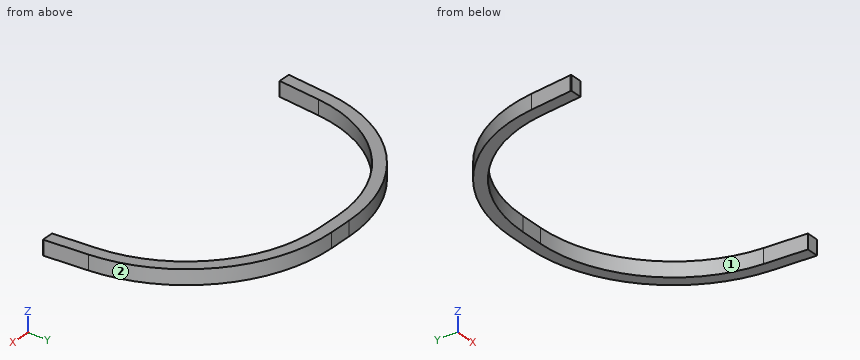
from build123d import *

# Parameters (mm, degrees)
EXTRUDE_1_DEPTH      = 5
SKETCH_3_W           = 25
SKETCH_3_H           = 3
SKETCH_3_W_2         = 27.5
CUT_EXTRUDE_1_DEPTH  = 396.82192966
SKETCH_2_R           = 1
CUT_EXTRUDE_2_DEPTH  = 396.82192966
SKETCH_4_R           = 1
CUT_EXTRUDE_3_DEPTH  = 396.82192966
SKETCH_5_W           = 3
SKETCH_5_H           = 20
CUT_EXTRUDE_4_DEPTH  = 396.82192966
SKETCH_6_W           = 52.963954937
SKETCH_6_H           = 5
SKETCH_6_W_2         = 50.247879271
CUT_EXTRUDE_5_DEPTH  = 396.82192966
SKETCH_7_W           = 24.499878537
SKETCH_7_H           = 5
SKETCH_7_W_2         = 25.63433041
SKETCH_7_W_3         = 30.65568147
SKETCH_7_W_4         = 13.75
CUT_EXTRUDE_6_DEPTH  = 396.82192966
CUT_EXTRUDE_10_DEPTH = 396.82192966
SKETCH_12_W          = 10
SKETCH_12_H          = 114.036005351
CUT_EXTRUDE_11_DEPTH = 396.82192966
SKETCH_13_W          = 5
SKETCH_13_H          = 15
EXTRUDE_2_DEPTH      = 3
CUT_EXTRUDE_12_DEPTH = 396.82192966
FILLET_1_R           = 45
CUT_EXTRUDE_13_DEPTH = 396.82192966


with BuildPart() as part:
    # 草图1 → 凸台-拉伸1 (new body)
    with BuildSketch(Plane.XY):
        Polygon((0, 0), (0, 85), (110, 105), (125, 175), (355, 175), (355, 0), (317.5, 0), (317.5, 5), (312.5, 60), (222.5, 60), (217.5, 5), (217.5, 0), (137.5, 0), (137.5, 5), (132.5, 60), (42.5, 60), (37.5, 5), (37.5, 0), align=None)
    extrude(amount=EXTRUDE_1_DEPTH)

    # 草图3 → 切除-拉伸1 (cut, through all)
    with BuildSketch(Plane.XY.offset(5)):
        with Locations((180, 173.5)):
            Rectangle(SKETCH_3_W, SKETCH_3_H)
        with Locations((341.25, 173.5)):
            Rectangle(SKETCH_3_W_2, SKETCH_3_H)
        with Locations((220, 173.5)):
            Rectangle(SKETCH_3_W, SKETCH_3_H)
        with Locations((260, 173.5)):
            Rectangle(SKETCH_3_W, SKETCH_3_H)
        with Locations((300, 173.5)):
            Rectangle(SKETCH_3_W, SKETCH_3_H)
        Polygon((152.5, 175), (152.5, 172), (124.357142857, 172), (125, 175), align=None)
    extrude(amount=-CUT_EXTRUDE_1_DEPTH, mode=Mode.SUBTRACT)

    # 草图2 → 切除-拉伸2 (cut, through all)
    with BuildSketch(Plane.XY.offset(5)):
        with Locations((200, 173)):
            Circle(SKETCH_2_R)
        with Locations((240, 173)):
            Circle(SKETCH_2_R)
        with Locations((280, 173)):
            Circle(SKETCH_2_R)
        with Locations((320, 173)):
            Circle(SKETCH_2_R)
        with Locations((160, 173)):
            Circle(SKETCH_2_R)
    extrude(amount=-CUT_EXTRUDE_2_DEPTH, mode=Mode.SUBTRACT)

    # 草图4 → 切除-拉伸3 (cut, through all)
    with BuildSketch(Plane.XY.offset(5)):
        with Locations((353, 162)):
            Circle(SKETCH_4_R)
        with Locations((353, 122)):
            Circle(SKETCH_4_R)
        with Locations((353, 82)):
            Circle(SKETCH_4_R)
        with Locations((353, 42)):
            Circle(SKETCH_4_R)
    extrude(amount=-CUT_EXTRUDE_3_DEPTH, mode=Mode.SUBTRACT)

    # 草图5 → 切除-拉伸4 (cut, through all)
    with BuildSketch(Plane.XY.offset(5)):
        with Locations((353.5, 142)):
            Rectangle(SKETCH_5_W, SKETCH_5_H)
        with Locations((353.5, 102)):
            Rectangle(SKETCH_5_W, SKETCH_5_H)
        with Locations((353.5, 62)):
            Rectangle(SKETCH_5_W, SKETCH_5_H)
        with Locations((353.5, 22)):
            Rectangle(SKETCH_5_W, SKETCH_5_H)
    extrude(amount=-CUT_EXTRUDE_4_DEPTH, mode=Mode.SUBTRACT)

    # 草图6 → 切除-拉伸5 (cut, through all)
    with BuildSketch(Plane.XY.offset(5)):
        with Locations((136.018022532, 2.5)):
            Rectangle(SKETCH_6_W, SKETCH_6_H)
        with Locations((217.623939635, 2.5)):
            Rectangle(SKETCH_6_W_2, SKETCH_6_H)
    extrude(amount=-CUT_EXTRUDE_5_DEPTH, mode=Mode.SUBTRACT)

    # 草图7 → 切除-拉伸6 (cut, through all)
    with BuildSketch(Plane.XY.offset(5)):
        with Locations((1.500060731, 2.5)):
            Rectangle(SKETCH_7_W, SKETCH_7_H)
        with Locations((36.567165205, 2.5)):
            Rectangle(SKETCH_7_W_2, SKETCH_7_H)
        with Locations((315.922159265, 2.5)):
            Rectangle(SKETCH_7_W_3, SKETCH_7_H)
        with Locations((348.125, 2.5)):
            Rectangle(SKETCH_7_W_4, SKETCH_7_H)
    extrude(amount=-CUT_EXTRUDE_6_DEPTH, mode=Mode.SUBTRACT)

    # 草图11 → 切除-拉伸10 (cut, through all)
    with BuildSketch(Plane.XY.offset(5)):
        Polygon((114.275152951, 110.632892707), (111.341745709, 111.261479973), (123.075374677, 166.018415161), (126.00878192, 165.389827895), align=None)
    extrude(amount=-CUT_EXTRUDE_10_DEPTH, mode=Mode.SUBTRACT)

    # 草图12 → 切除-拉伸11 (cut, through all)
    with BuildSketch(Plane.XY.offset(5)):
        with Locations((5, 77.018002676)):
            Rectangle(SKETCH_12_W, SKETCH_12_H)
    extrude(amount=-CUT_EXTRUDE_11_DEPTH, mode=Mode.SUBTRACT)

    # 草图13 → 凸台-拉伸2 (add)
    with BuildSketch(Plane.XY.offset(5)):
        with Locations((7.5, 37.5)):
            Rectangle(SKETCH_13_W, SKETCH_13_H)
        with Locations((7.5, 67.5)):
            Rectangle(SKETCH_13_W, SKETCH_13_H)
    extrude(amount=-EXTRUDE_2_DEPTH)

    # 草图15 → 切除-拉伸12 (cut, through all)
    with BuildSketch(Plane.XY.offset(5)):
        Polygon((35.491174943, 86.370968223), (34.596747752, 91.290317773), (19.838699101, 88.6070362), (20.733126292, 83.68768665), align=None)
        Polygon((54.274145954, 94.868026537), (55.168573145, 89.948676987), (69.926621797, 92.63195856), (69.032194606, 97.55130811), align=None)
        Polygon((88.709592808, 101.129016874), (89.604019999, 96.209667324), (104.36206865, 98.892948897), (103.467641459, 103.812298447), align=None)
    extrude(amount=-CUT_EXTRUDE_12_DEPTH, mode=Mode.SUBTRACT)

    # 圆角1
    fillet_1_edges = [part.edges().sort_by_distance(p)[0] for p in [
        (312.5, 60, 2.5),
        (222.5, 60, 2.5),
        (132.5, 60, 2.5),
        (42.5, 60, 2.5),
    ]]
    fillet(fillet_1_edges, radius=FILLET_1_R)

    # 草图16 → 切除-拉伸13 (cut, through all)
    with BuildSketch(Plane.XY.offset(5)):
        with BuildLine():
            Line((33.516427174, 5), (33.516427174, 5.362142984))
            Line((33.516427174, 5.362142984), (34.79589159, 19.436251556))
            ThreePointArc((34.79589159, 19.436251556), (50.552082583, 51.182705304), (83.594658707, 64))
            Line((83.594658707, 64), (91.405341293, 64))
            ThreePointArc((91.405341293, 64), (124.447917417, 51.182705304), (140.20410841, 19.436251556))
            Line((140.20410841, 19.436251556), (141.483572826, 5.362142984))
            Line((141.483572826, 5.362142984), (141.483572826, 5))
            Line((141.483572826, 5), (162.5, 0))
            Line((162.5, 0), (192.5, 0))
            Line((192.5, 0), (217.5, 5))
            Line((217.5, 5), (317.5, 5))
            Line((317.5, 5), (331.25, 0))
            Line((331.25, 0), (341.25, 0))
            Line((341.25, 0), (355, 5))
            Line((355, 5), (355, 172))
            Line((355, 172), (327.5, 175))
            Line((327.5, 175), (152.5, 175))
            Line((152.5, 175), (124.357142857, 172))
            Line((124.357142857, 172), (88.709592808, 101.129016874))
            Line((88.709592808, 101.129016874), (10, 86.818181818))
            Line((10, 86.818181818), (5, 75))
            Line((5, 75), (0, 20))
            Line((0, 20), (0, 5))
            Line((0, 5), (13.75, 0))
            Line((13.75, 0), (23.75, 0))
            Line((23.75, 0), (33.516427174, 5))
        make_face()
    extrude(amount=-CUT_EXTRUDE_13_DEPTH, mode=Mode.SUBTRACT)


solid = part.part
Geometry: final body of the model. Coordinates: model frame, mm. Face numbers are marked on the shaded views. Round coordinates to 2 decimals unless told otherwise and drop trailing zeros. Loops run counter-clockwise (first coordinate to the right, second up) from the corner with the lowest first, then second, coordinate; pieces in that order, holes last. Notation, with made-up numbers: (-20.5, 38.25) - (1.5, 38.25) arc R31 cw to (1.5, 77.25) - close; hole circle Ø2 at (6, 60). An arc over 180 degrees is marked (long way). Write each question's results on one line, items separated by ' | '. Start each with the question number.
1) Mould query, pull axis X, two halves, no side actions, for the marked faces 1 and 2. Classes: released by +X, released by -X, zero draft, split by the parting line, or undercut.
2) Line query: probe 1 along X at (y, z) = (13.5, 1.35); probe 2 along X at (y, z) = (8, 3.85); probe 3 along Y at (x, z) = (83.5, 2.6). Output: solid intervals per line, ascending. Write a range as [from, to].
3) First-contact query: P1, Ø2, axis at y = 20.5, z = 1.5, coming from the -X side; P2, Ø3, axis at y = 39.5, z = 4, coming from the -X side; P3, Ø2, axis at y = 33, z = 4.5, coming from the -X side. Flat tips, straight axial feed; report the tip coordinate or a pass-through.
4) Cut plane D-D on x = 62.5. Return loops of the section in (y, z).
5) Cut plane C-C on y = 53. Return loops of the section in (x, z), then the cut area to 3 significant figures.
6) Cut plane B-B on z = 2.15. Return loops of the section in (x, y), then the cut area to 3 significant figures.
7) Cut plane A-A on y = 40.5. Return loops of the section in (x, z), then the cut area to 3 significant figures.
Verdict:
1) face 1: undercut | face 2: released by +X
2) probe 1: x = [34.26, 38.27], [136.73, 140.74] | probe 2: x = [33.76, 37.77], [137.23, 141.24] | probe 3: y = [60, 64]
3) P1: stops at x = 34.8 | P2: stops at x = 40.33 | P3: stops at x = 37.64
4) outline: (54.75, 0) - (59.23, 0) - (59.23, 5) - (54.75, 5) - close
5) outline: (52.66, 0) - (59.49, 0) - (59.49, 5) - (52.66, 5) - close; (115.51, 0) - (122.34, 0) - (122.34, 5) - (115.51, 5) - close | area: 68.3 mm2
6) outline: (33.52, 5) - (37.5, 5) - (38.78, 19.07) arc R45 cw to (83.59, 60) - (91.41, 60) arc R45 cw to (136.22, 19.07) - (137.5, 5) - (141.48, 5) - (141.48, 5.36) - (140.2, 19.44) arc R49 ccw to (91.41, 64) - (83.59, 64) arc R49 ccw to (34.8, 19.44) - (33.52, 5.36) - close | area: 702 mm2
7) outline: (41.75, 0) - (46.52, 0) - (46.52, 5) - (41.75, 5) - close; (128.48, 0) - (133.25, 0) - (133.25, 5) - (128.48, 5) - close | area: 47.6 mm2
